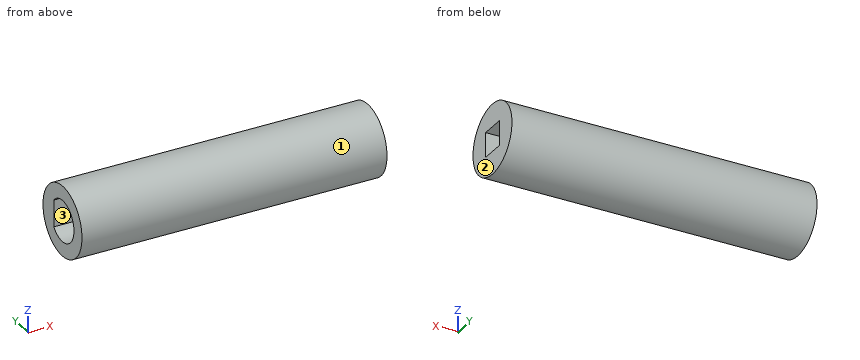
Autodesk Inventor part; units mm, degrees
ref_plane "YZ Plane" through (0, 0, 0) normal (1, 0, 0) x (0, 1, 0)
ref_plane "XZ Plane" through (0, 0, 0) normal (0, 1, 0) x (-1, 0, 0)
ref_plane "XY Plane" through (0, 0, 0) normal (0, 0, 1) x (1, 0, 0)
sketch "Sketch1" plane through (0, 0, 0) normal (1, 0, 0) x (0, 1, 0)
  circle A0 centre (0, 0) radius 5.3975
  circle A1 centre (0, 0) radius 3.175
  line L0 (-3.175, 0) -> (2.413, 0) construction
  line L1 (2.413, 0) -> (2.413, -2.0635)
  line L2 (2.413, 0) -> (2.413, 2.0635)
  dimension "d0" = 10.795
  dimension "d1" = 6.35
  dimension "d2" = 5.588
extrude "Extrusion1" add sketch "Sketch1" along normal blind 25.4 contours A0 | A1 L1 L2 picked at (2.5514, -1.1687)
sketch "Sketch2" plane through (25.4, 0, 0) normal (1, 0, 0) x (0, 0, -1)
  circle A0 centre (0, 0) radius 5.3975
  dimension "d11" = 10.795
extrude "Extrusion2" add sketch "Sketch2" along normal blind 2.54
sketch "Sketch3" plane through (27.94, 0, 0) normal (1, 0, 0) x (0, 0, -1)
  arc A0 (-2.0635, 2.413) -> (2.0635, 2.413) centre (0, 0) ccw
  circle A1 centre (0, 0) radius 5.3975
  line L0 (1.905, -1.905) -> (-1.905, -1.905)
  line L1 (-1.905, -1.905) -> (-1.905, 1.905)
  line L2 (-1.905, 1.905) -> (1.905, 1.905)
  line L3 (1.905, 1.905) -> (1.905, -1.905)
  line L4 (1.905, -1.905) -> (-1.905, 1.905) construction
  line L5 (-1.905, -1.905) -> (1.905, 1.905) construction
  dimension "d7" = 3.81
  dimension "d8" = 3.81
  dimension "d12" = 10.795
extrude "Extrusion3" add sketch "Sketch3" along normal blind 19.05
properties part number "NeveRestVex"
Geometry: final body of the model. Coordinates: model frame, mm. Face numbers are marked on the shaded views. Round coordinates to 2 decimals unless told otherwise and drop trailing zeros. Order: outer loops, then holes, each group sorted by start corner. A loop starts at its lowest first (then second) coordinate and runs counter-clockwise, first axis right, second up. Notation, with made-up numbers: M 15.5,7 L 74.5,7 A23 cw 74.5,31 Z; hole C 85.5,-9.75 d11. An arc over 180 degrees is marked long. One line per item, written item: value.
(1) Line query: probe 1 along Y at (x, z) = (17.75, 0) (1 decimal); probe 2 along Z at (x, y) = (11.5, 0) (1 decimal); probe 3 along X at (y, z) = (0.5, -1.25). Output: solid intervals per line, ascending. Write a range as [from, to].
Result sheet:
probe 1: [-5.4, -3.2], [2.4, 5.4]
probe 2: [-5.4, -3.2], [3.2, 5.4]
probe 3: [25.4, 27.94]
(2) Cut plane D-D (y = -3.75). Return the cut outline in (x, z).
Result sheet:
outline: M 0,-3.88 L 46.99,-3.88 L 46.99,3.88 L 0,3.88 Z
(3) Cut plane C-C (x = 27.5). Return the cut outline in (y, z) (1 decimal).
Result sheet:
outline: C 0,0 d10.8
(4) Cut plane A-A (x = 33). Return the cut outline in (y, z) (1 decimal).
Result sheet:
outline: C 0,0 d10.8; hole M -1.9,-1.9 L 1.9,-1.9 L 1.9,1.9 L -1.9,1.9 Z
(5) Pin query (flat end, axial travel): P1, Ø4, axis at x = 40, z = 3, coming from the +Y side; P2, Ø3, axis at x = 18, z = 3.5, coming from the -Y side; P3, Ø1.5, axis at x = 8, z = 1, coming from the -Y side. Return the tip coordinate at first contact, or that it passes through.
Result sheet:
P1: y = 5.3
P2: y = -5.01
P3: y = -5.39
(6) Cut plane B-B (z = 1.5). Return the cut outline in (x, y) (3 decimals), and give its area (3 significant figures).
Result sheet:
outline: M 0,-5.185 L 46.99,-5.185 L 46.99,-1.905 L 27.94,-1.905 L 27.94,1.905 L 46.99,1.905 L 46.99,5.185 L 0,5.185 L 0,2.413 L 25.4,2.413 L 25.4,-2.798 L 0,-2.798 Z
area: 282 mm2
(7) Pull-direction query (Z, two-part tool) for the marked faces 1, 2 and 3; classes: pulls with the +Z half, pulls with the -Z half, needs draft (parallel to the pull), parting line crosses it, or undercut.
Result sheet:
face 1: parting line crosses it
face 2: needs draft
face 3: undercut
